Design review of the part built by this model. Coordinates are the model's own, in mm. A direction names the side the tool comes from. Give positions to 0.01 mm unless a question says otherwise; leave off trailing zeros. Loops run counter-clockwise (first coordinate to the right, second up) from the corner with the lowest first, then second, coordinate; pieces in that order, holes last. Notation, with made-up numbers: (89.25, -14.75) -> (98.25, -14.75) arc R34 ccw to (98.25, 17.25) -> close; hole circle Ø6 at (2.25, 51). An arc over 180 degrees is marked (long way). Use CSV: the item, a comma, the result in double quotes. Start each with the question number.
Item 1: We need section A-A (x = -281). State the section outline as (y, z) points, plus the area to 3 significant figures.
Item 2: We need section D-D (y = -350.5). State the section outline as (x, z) points, plus the area to 3 significant figures.
Item 3: We need section C-C (z = 316.5). State the section outline as (x, y) points, plus the area to 3 significant figures.
Item 4: We need section B-B (x = -259). State the section outline as (y, z) points.
Item 5: For faces 4 (the face through (-301.276, -291.131, 225.915)), 5 (the face through (-250.6, -395.36, 261.55)), 6 (the face through (-308.33, -258.99, 200.6)), 7 (the face through (-277.29, -496.57, 385.99)), list the 3-axis set-ups (+Z, -Z, +X, -X, +Y, -Y) from which the entire face can be reached by the end or side of a thin tool; tool diameter is ignored.
Item 6: Wall thickness on line 1 along Z through (x, y) = (-247.5, -445.5); line 2 along Z through (x, y) = (-236, -508); line 3 along X through (y, z) = (-381.5, 276.5): over which ranges is each line inside the solid? List them lowest first. Write a range as from..to.
Item 7: Clearance check with flat-ended pins moving along their axes: pin 1 (8 mm diameter, centred on x = -258.5, z = 358.5, fed in from +Y); pin 2 (4 mm diameter, centred on x = -289, y = -346.5, fed in from -Z); pin 3 (12 mm diameter, centred on x = -235.5, y = -296.5, fed in from -Z). State where each tip first meets the part, or that it passes through.
Item 8: The part is to be moulded in two halves that separate along X. For faces 1 (the face through (-308.838, -317.138, 246.079)), 2 (the face through (-272.834, -346.333, 269.541)), 3 (the face through (-263, -241.721, 152)), say which applies: +X half, -X half, draft (parallel to the pull), parting line (faces both ways), or undercut.
from build123d import *

# Parameters (mm, degrees)
BOSS_EXTRUDE1_DEPTH    = 2.54
SKETCH3_W              = 635
SKETCH3_H              = 1270
BOSS_EXTRUDE2_DEPTH    = 2.54
CUT_EXTRUDE1_START     = -114.3
CUT_EXTRUDE1_OUTLINE_W = 635
CUT_EXTRUDE1_OUTLINE_H = 1004
CUT_EXTRUDE1_DEPTH     = 896.190073664


# Read off the part's stored shape, not the designer's step: Cut-Extrude1
with BuildPart() as part:
    # Sketch2 → Boss-Extrude1 (new body)
    with BuildSketch(Plane(origin=(0, 0, 0), x_dir=(1, 0, 0), z_dir=(0, 1, 0))):
        with BuildLine():
            Line((-190.5, 0), (190.5, 0))
            Line((190.5, 0), (172.589792707, 64.649970609))
            ThreePointArc((172.589792707, 64.649970609), (148.320865378, 100.476994518), (107.315, 114.3))
            Line((107.315, 114.3), (-107.315, 114.3))
            ThreePointArc((-107.315, 114.3), (-148.320865378, 100.476994518), (-172.589792707, 64.649970609))
            Line((-172.589792707, 64.649970609), (-190.5, 0))
        make_face()
    extrude(amount=-BOSS_EXTRUDE1_DEPTH)

    # Sketch3 → Boss-Extrude2 (add)
    with BuildSketch(Plane(origin=(0, 0, 0), x_dir=(1, 0, 0), z_dir=(0, 0.6156614753256567, 0.7880107536067232))):
        with Locations((0, -635)):
            Rectangle(SKETCH3_W, SKETCH3_H)
    extrude(amount=-BOSS_EXTRUDE2_DEPTH)

    # Cut-Extrude1 outline → Cut-Extrude1 (cut)
    with BuildSketch(Plane.XY.offset(CUT_EXTRUDE1_START)):
        with Locations((0, -502)):
            Rectangle(CUT_EXTRUDE1_OUTLINE_W, CUT_EXTRUDE1_OUTLINE_H)
        with BuildLine():
            Line((-236.906583619, -241.721009662), (-190.5, -571.921009662))
            Line((-190.5, -571.921009662), (-266.7, -571.921009662))
            Line((-266.7, -571.921009662), (-294.096224924, -376.98674033))
            ThreePointArc((-294.096224924, -376.98674033), (-272.877245274, -346.141774354), (-305.43807978, -327.663433526))
            Line((-305.43807978, -327.663433526), (-312.269080611, -306.514247899))
            ThreePointArc((-312.269080611, -306.514247899), (-301.277723529, -291.035795076), (-312.982021819, -276.089162217))
            Line((-312.982021819, -276.089162217), (-303.634542969, -241.721009662))
            Line((-303.634542969, -241.721009662), (-236.906583619, -241.721009662))
        make_face(mode=Mode.SUBTRACT)
    extrude(amount=CUT_EXTRUDE1_DEPTH, mode=Mode.SUBTRACT)

    # Sweep1: sweep along a curve in space
    with BuildLine() as sweep1_path:
        Line((-236.906583619, -241.721009662, 185.629844207), (-190.5, -571.921009662, 443.61035808))
    # Sketch8 → Sweep1 (sweep)
    with BuildSketch(Plane(origin=(0, -241.721009662, 0), x_dir=(1, 0, 0), z_dir=(0, 1, 0))):
        Polygon((-236.906583619, -185.629844207), (-310.929097821, -84.029844207), (-312.982021819, -85.525539048), (-240.049223095, -185.629844207), align=None)
    sweep(path=sweep1_path.line)


solid = part.part
Results found:
1,outline,"(-470.17, 364.11) -> (-371.03, 286.66) -> (-371.03, 289.88) -> (-470.17, 367.34) -> close; (-469.28, 263.32) -> (-454.68, 250.41) -> (-241.72, 125.11) -> (-241.72, 129.42) -> close; (-332.64, 256.66) -> (-241.72, 185.63) -> (-241.72, 188.85) -> (-332.64, 259.88) -> close"
1,area,"1,560 mm²"
2,outline,"(-297.69, 170.51) -> (-295.64, 169.02) -> (-221.62, 270.62) -> (-221.62, 273.84) -> (-272.27, 273.84) -> (-272.27, 270.62) -> (-224.76, 270.62) -> close"
2,area,"480 mm²"
3,outline,"(-290.14, -405.1) -> (-289.57, -409.23) -> (-216.51, -409.23) -> (-271.43, -537.35) -> (-269.11, -539.27) -> (-213.37, -409.23) -> (-213.94, -405.1) -> close"
3,area,"720 mm²"
4,outline,"(-571.92, 349.59) -> (-241.72, 155.31) -> (-241.72, 159.62) -> (-571.92, 353.9) -> close; (-571.92, 443.61) -> (-241.72, 185.63) -> (-241.72, 188.85) -> (-571.92, 446.83) -> close"
5,face 4,"+Z, -X"
5,face 5,"-X"
5,face 6,"+Z, -X, +Y"
5,face 7,"+Z, -Z, -X, -Y"
6,line 1,"290.99..295.3, 344.84..348.06"
6,line 2,"343.55..347.86, 393.67..396.89"
6,line 3,"-233.76..-230.62"
7,pin 1,"y = -453.74"
7,pin 2,"z = 172.79"
7,pin 3,"z = 210.83"
8,face 1,"-X half"
8,face 2,"undercut"
8,face 3,"draft"
